Here's how the part is built. I have some questions about the finished solid (model axes, mm). Face numbers are marked on the shaded views. A direction names the side the tool comes from. Coordinates: 2 decimals unless noted, no trailing zeros. Write each loop counter-clockwise with the first axis right and the second up, starting at its lowest first coordinate (ties: lowest second). Pieces come first, ordered by that corner, then holes.
Item 1: If we section it at B-B (y = 6): Please give me the cut outline in (x, z), then the cut area to 3 significant figures.
Item 2: We'd pull the mould along X, two halves only. Please class the marked faces 4, 5, 6 and 7: +X half, -X half, draft (parallel to the pull), parting line (faces both ways), or undercut.
Item 3: If we section it at A-A (z = 23.5): Please give me the cut outline in (x, y), then the cut area to 3 significant figures.
Item 4: If I drill on line 1 (Y direction, x = 18.5, z = -23.5); line 2 (Z direction, x = 9.5, y = 5.5); line 3 (X direction, y = 11.25, z = -18), over which ranges is the centre line in solid material (lowest first)?
Item 5: For the marked faces 1, 2 and 3, which set-ups out of +Z, -Z, +X, -X, +Y, -Y let a thin tool reach every point of the face, with its end or its side?
Item 6: If we section it at D-D (y = 2.25): Please give me the cut outline in (x, z), then the cut area to 3 significant figures.
Item 7: I'm going to push flat-ended pins straight in: pin 1 Ø3 at (y, z) = (6, -23.5) entering from +X; pin 2 Ø3 at (x, y) = (-8, 5) entering from -Z. Where does each tip first touch, or does it pass through?
Item 8: If we section it at C-C (x = -19): Please give me the cut outline in (y, z).
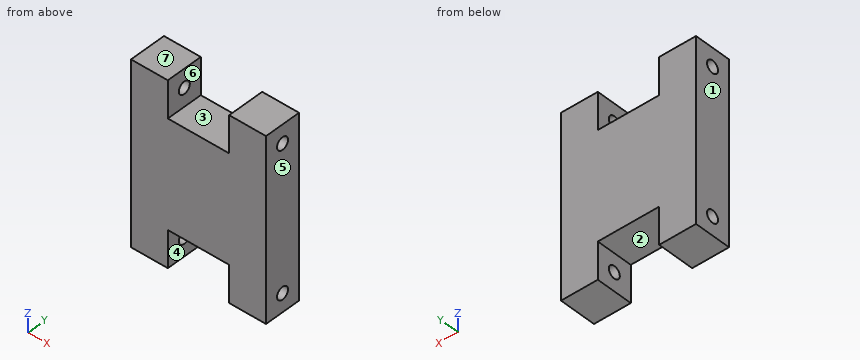
from build123d import *

# Parameters (mm, degrees)
SKETCH1_W           = 44
SKETCH1_H           = 59
BOSS_EXTRUDE1_DEPTH = 12
CUT_EXTRUDE1_REACH  = 40.707
SKETCH2_W           = 20
SKETCH2_H           = 12
CUT_EXTRUDE2_REACH  = 56.316
SKETCH3_R           = 2


with BuildPart() as part:
    # Sketch1 → Boss-Extrude1 (new body)
    with BuildSketch(Plane(origin=(0, 0, 0), x_dir=(1, 0, 0), z_dir=(0, 1, 0))):
        Rectangle(SKETCH1_W, SKETCH1_H)
    extrude(amount=BOSS_EXTRUDE1_DEPTH)

    # Sketch2 → Cut-Extrude1 (cut, up to next)
    with BuildSketch(Plane(origin=(0, 12, 0), x_dir=(1, 0, 0), z_dir=(0, 1, 0)), mode=Mode.PRIVATE) as cut_extrude1_sk1:
        with Locations((0, 23.5)):
            Rectangle(SKETCH2_W, SKETCH2_H)
    cut_extrude1_tool1 = extrude(cut_extrude1_sk1.sketch, amount=-CUT_EXTRUDE1_REACH, mode=Mode.PRIVATE) & part.part
    # Sketch2 → Cut-Extrude1 (cut, up to next)
    with BuildSketch(Plane(origin=(0, 12, 0), x_dir=(1, 0, 0), z_dir=(0, 1, 0)), mode=Mode.PRIVATE) as cut_extrude1_sk2:
        with Locations((0, -23.5)):
            Rectangle(SKETCH2_W, SKETCH2_H)
    cut_extrude1_tool2 = extrude(cut_extrude1_sk2.sketch, amount=-CUT_EXTRUDE1_REACH, mode=Mode.PRIVATE) & part.part
    add(cut_extrude1_tool1.solids().sort_by_distance((0, 12, -23.5))[0], mode=Mode.SUBTRACT)
    add(cut_extrude1_tool2.solids().sort_by_distance((0, 12, 23.5))[0], mode=Mode.SUBTRACT)

    # Cut-Extrude2: up to this face of the body (flat: up to its plane)
    cut_extrude2_end = Plane(part.part.faces().sort_by_distance((22, 6, 0))[0])
    # Sketch3 → Cut-Extrude2 (cut, up to the picked face)
    with BuildSketch(Plane.ZY.offset(22), mode=Mode.PRIVATE) as cut_extrude2_sk1:
        with Locations((-23.5, 6)):
            Circle(SKETCH3_R)
    cut_extrude2_tool1 = split(extrude(cut_extrude2_sk1.sketch, amount=-CUT_EXTRUDE2_REACH, mode=Mode.PRIVATE), bisect_by=cut_extrude2_end, keep=Keep.BOTH, mode=Mode.PRIVATE)
    cut_extrude2 = cut_extrude2_tool1.solids().sort_by(Axis((-22, 6, -23.5), (1, 0, 0)))[0]
    add(cut_extrude2, mode=Mode.SUBTRACT)

    # Mirror1: Cut-Extrude2 across plane
    add(cut_extrude2.mirror(Plane.XY), mode=Mode.SUBTRACT)


solid = part.part
Answer list:
1. outline: (-22, -29.5) - (-10, -29.5) - (-10, -25.5) - (-22, -25.5) - close; (-22, -21.5) - (-10, -21.5) - (-10, -17.5) - (10, -17.5) - (10, -21.5) - (22, -21.5) - (22, 21.5) - (10, 21.5) - (10, 17.5) - (-10, 17.5) - (-10, 21.5) - (-22, 21.5) - close; (-22, 25.5) - (-10, 25.5) - (-10, 29.5) - (-22, 29.5) - close; (10, -29.5) - (22, -29.5) - (22, -25.5) - (10, -25.5) - close; (10, 25.5) - (22, 25.5) - (22, 29.5) - (10, 29.5) - close
1. area: 1,920 mm2
2. face 4: undercut
2. face 5: +X half
2. face 6: undercut
2. face 7: draft
3. outline: (-22, 0) - (-10, 0) - (-10, 4) - (-22, 4) - close; (-22, 8) - (-10, 8) - (-10, 12) - (-22, 12) - close; (10, 0) - (22, 0) - (22, 4) - (10, 4) - close; (10, 8) - (22, 8) - (22, 12) - (10, 12) - close
3. area: 192 mm2
4. line 1: y = 0 to 4, 8 to 12
4. line 2: z = -17.5 to 17.5
4. line 3: x = -22 to -10, 10 to 22
5. face 1: +Z, -Z, -X, +Y, -Y
5. face 2: -Z, +Y, -Y
5. face 3: +Z, +Y, -Y
6. outline: (-22, -29.5) - (-10, -29.5) - (-10, -17.5) - (10, -17.5) - (10, -29.5) - (22, -29.5) - (22, 29.5) - (10, 29.5) - (10, 17.5) - (-10, 17.5) - (-10, 29.5) - (-22, 29.5) - close
6. area: 2,120 mm2
7. pin 1: passes through
7. pin 2: stops at z = -17.5
8. outline: (0, -29.5) - (12, -29.5) - (12, 29.5) - (0, 29.5) - close; hole circle Ø4 at (6, -23.5); hole circle Ø4 at (6, 23.5)
